Geometry check sheet. Reference: the model listing, model coordinates, mm. A direction names the side the tool comes from. Coordinates: 2 decimals unless noted, no trailing zeros. Order: outer loops, then holes, each group sorted by start corner. A loop starts at its lowest first (then second) coordinate and runs counter-clockwise, first axis right, second up. Notation, with made-up numbers: (-23.75, 69.25) - (-16.75, 69.25) arc R33 cw to (-16.75, 101.25) - close; hole circle Ø1 at (51.25, -30). An arc over 180 degrees is marked (long way). Use CSV: the item, a comma, the result in double quotes. Start each with the question number.
1) Thickness scan on probe 1 along Z at (x, y) = (0, 21); probe 2 along X at (y, z) = (245, -116); probe 3 along X at (y, z) = (12, -35). Record the ranges inside material, lowest first. Write a range as [from, to].
2) Sectioned sample at D-D, the plane x = 0. Count the separate pieces of the cut face and the enclosed holes in it, and give its area (3 significant figures).
3) Sectioned sample at A-A, the plane z = -35. Record the cut outline in (x, y).
4) Draft check along X on faces 1 (the cylindrical face through (-0.77, 174.19, -139.99)), 2 (the flat face through (0, 95, -125)), 3 (the flat face through (0, 245, -125)), 4 (the flat face through (-7.5, 119, -176)). Enter one of: released by +X, released by -X, zero draft, split by the parting line, or undercut.
5) Tool access check on faces 5 (the cylindrical face through (17.64, 236.695, -175.928)), 6 (the cylindrical face through (-17.36, 251.76, -128.36)), 7 (the cylindrical face through (-7.509, 32.465, -58.846)). Record the directions out of +Z, -Z, +X, -X, +Y, -Y that give a thin tool (end or side, any length) a straight path to the whole face; none if there is none.
6) Sectioned sample at C-C, the plane y = 20. Record the cut outline in (x, z), and give its area (3 significant figures).
7) Depth check by flat-ended pin: P1, Ø2, axis at x = -37.5, z = -153.5, coming from the +Y side; P2, Ø3, axis at y = 136, z = -186, coming from the +X side; P3, Ø12, axis at x = 25, y = 93.5, coming from the -Z side. Enter the tip coordinate at first touch or a pass-through.
8) Sectioned sample at B-B, the plane x = -44. Record the cut outline in (y, z), and give its area (3 significant figures).
from build123d import *

# Parameters (mm, degrees)
BOSS_EXTRUDE1_DEPTH     = 50
BOSS_EXTRUDE4_DEPTH     = 55
BOSS_EXTRUDE5_DEPTH     = 27.5
CUT_EXTRUDE1_DEPTH      = 20
FILLET1_R               = 13
FILLET2_R               = 25
FILLET3_R               = 10
FILLET4_R               = 20
CUT_EXTRUDE2_DEPTH      = 461.353125329
CUT_EXTRUDE2_DEPTH_BACK = 461.353125329
CUT_EXTRUDE3_START      = -110
SKETCH14_W              = 10
SKETCH14_H              = 90
CUT_EXTRUDE3_DEPTH      = 110
SKETCH15_R              = 25
BOSS_EXTRUDE6_DEPTH     = 5
LPATTERN1_COUNT         = 2
LPATTERN1_PITCH         = 290
HOLE1_D                 = 20
HOLE2_D                 = 16
HOLE2_DEPTH             = 25
LPATTERN2_COUNT         = 2
LPATTERN2_PITCH         = 150


with BuildPart() as part:
    # Sketch2 → Boss-Extrude1 (new, symmetric)
    with BuildSketch(Plane(origin=(0, 0, 0), x_dir=(0, 0, -1), z_dir=(1, 0, 0))):
        Polygon((0, 0), (360, 0), (360, 30), (125, 30), (125, 265), (100, 265), (100, 30), (0, 30), align=None)
    extrude(amount=BOSS_EXTRUDE1_DEPTH, both=True)

    # Sketch7 → Boss-Extrude4 (add, symmetric)
    with BuildSketch(Plane(origin=(0, 0, 0), x_dir=(0, 0, -1), z_dir=(1, 0, 0))):
        with BuildLine():
            Line((100, 225), (100, 125))
            ThreePointArc((100, 125), (150, 175), (100, 225))
        make_face()
    extrude(amount=BOSS_EXTRUDE4_DEPTH, both=True)

    # Sketch11 → Boss-Extrude5 (add, symmetric)
    with BuildSketch(Plane(origin=(0, 0, 0), x_dir=(0, 0, -1), z_dir=(1, 0, 0))):
        with BuildLine():
            Line((209.572335871, 205.781812899), (273.551683491, 30))
            Line((273.551683491, 30), (125, 30))
            Line((125, 30), (125, 265))
            ThreePointArc((125, 265), (176.621879272, 248.723683986), (209.572335871, 205.781812899))
        make_face()
    extrude(amount=BOSS_EXTRUDE5_DEPTH, both=True)

    # Sketch12 → Cut-Extrude1 (cut)
    with BuildSketch(Plane(origin=(27.5, 0, 0), x_dir=(0, 0, -1), z_dir=(1, 0, 0))):
        with BuildLine():
            Line((125, 255), (125, 218.301270189))
            ThreePointArc((125, 218.301270189), (150, 175), (125, 131.698729811))
            Line((125, 131.698729811), (125, 30))
            Line((125, 30), (262.909905767, 30))
            Line((262.909905767, 30), (200.175409663, 202.361611466))
            ThreePointArc((200.175409663, 202.361611466), (170.886114908, 240.532163543), (125, 255))
        make_face()
    cut_extrude1 = extrude(amount=-CUT_EXTRUDE1_DEPTH, mode=Mode.SUBTRACT)

    # Mirror1: Cut-Extrude1 across plane
    add(cut_extrude1.mirror(Plane(origin=(0, 0, 0), x_dir=(0, 0, 1), z_dir=(1, 0, 0))), mode=Mode.SUBTRACT)

    # Fillet1
    fillet1_edges = [part.edges().sort_by_distance(p)[0] for p in [
        (17.5, 30, -262.909905767),
        (-17.5, 30, -262.909905767),
    ]]
    fillet(fillet1_edges, radius=FILLET1_R)

    # Fillet2
    fillet2_edges = [part.edges().sort_by_distance(p)[0] for p in [
        (0, 30, -273.551683491),
    ]]
    fillet(fillet2_edges, radius=FILLET2_R)

    # Fillet3
    fillet3_edges = [part.edges().sort_by_distance(p)[0] for p in [
        (17.5, 255, -125),
        (-17.5, 255, -125),
    ]]
    fillet(fillet3_edges, radius=FILLET3_R)

    # Fillet4
    fillet4_edges = [part.edges().sort_by_distance(p)[0] for p in [
        (0, 30, -100),
        (28.75, 30, -125),
        (-28.75, 30, -125),
    ]]
    fillet(fillet4_edges, radius=FILLET4_R)

    # Sketch13 → Cut-Extrude2 (cut, two sides: drawn at the far end of the back side and taken through both)
    with BuildSketch(Plane(origin=(55, 0, 0), x_dir=(0, 0, -1), z_dir=(1, 0, 0)).offset(-CUT_EXTRUDE2_DEPTH_BACK)):
        with BuildLine():
            Line((100, 215), (100, 135))
            ThreePointArc((100, 135), (140, 175), (100, 215))
        make_face()
    extrude(amount=CUT_EXTRUDE2_DEPTH + CUT_EXTRUDE2_DEPTH_BACK, mode=Mode.SUBTRACT)

    # Sketch14 → Cut-Extrude3 (cut)
    with BuildSketch(Plane(origin=(55, 0, 0), x_dir=(0, 0, -1), z_dir=(1, 0, 0)).offset(CUT_EXTRUDE3_START)):
        with Locations((100, 175)):
            Rectangle(SKETCH14_W, SKETCH14_H)
    extrude(amount=CUT_EXTRUDE3_DEPTH, mode=Mode.SUBTRACT)

    # Sketch15 → Boss-Extrude6 (add)
    with BuildSketch(Plane(origin=(0, 30, 0), x_dir=(1, 0, 0), z_dir=(0, 1, 0))):
        with Locations(Location((0, 35, 0), (0, 0, 90))):
            Circle(SKETCH15_R)
    boss_extrude6 = extrude(amount=BOSS_EXTRUDE6_DEPTH)

    # LPattern1: Boss-Extrude6 ×2
    with Locations(*[(0, 0, -i * LPATTERN1_PITCH) for i in range(1, LPATTERN1_COUNT)]):
        add(boss_extrude6)

    # Hole1 (through all)
    with Locations(Plane(origin=(0, 35, 0), x_dir=(1, 0, 0), z_dir=(0, 1, 0))):
        with Locations((0, 35), (0, 325)):
            Hole(HOLE1_D / 2)

    # Hole2
    with Locations(Plane.XY.offset(-100)):
        with Locations((0, 245)):
            hole2 = Hole(HOLE2_D / 2, depth=HOLE2_DEPTH)

    # LPattern2: Hole2 ×2
    with Locations(*[(0, -i * LPATTERN2_PITCH, 0) for i in range(1, LPATTERN2_COUNT)]):
        add(hole2, mode=Mode.SUBTRACT)


solid = part.part
Evaluation:
1,probe 1,"[-360, -335], [-315, -45], [-25, 0]"
1,probe 2,"[-50, -8], [8, 50]"
1,probe 3,"[-50, -10], [10, 50]"
2,separate pieces,"3"
2,enclosed holes,"0"
2,area,"36,700 mm²"
3,outline,"(-50, 0) - (-10, 0) - (-10, 35) - (-25, 35) - (-25, 30) - (-50, 30) - close; (10, 0) - (50, 0) - (50, 30) - (25, 30) - (25, 35) - (10, 35) - close"
4,face 1,"zero draft"
4,face 2,"undercut"
4,face 3,"undercut"
4,face 4,"released by -X"
5,face 5,"+X"
5,face 6,"-X"
5,face 7,"+Y"
6,outline,"(-50, -360) - (50, -360) - (50, 0) - (-50, 0) - close; hole circle Ø20 at (0, -325); hole circle Ø20 at (0, -35)"
6,area,"35,400 mm²"
7,P1,"y = 30"
7,P2,"x = 7.5"
7,P3,"z = -252.62"
8,outline,"(0, -360) - (30, -360) - (30, -145) arc R20 cw to (50, -125) - (131.7, -125) arc R50 ccw to (218.3, -125) - (265, -125) - (265, -100) - (220, -100) - (220, -105) - (214.69, -105) arc R40 cw to (135.31, -105) - (130, -105) - (130, -100) - (50, -100) arc R20 cw to (30, -80) - (30, 0) - (0, 0) - close"
8,area,"15,800 mm²"
